Geometry: final body of the model. Coordinates: model frame, mm. A direction names the side the tool comes from. Give positions to 0.01 mm unless a question says otherwise; leave off trailing zeros. Write each loop counter-clockwise with the first axis right and the second up, starting at its lowest first coordinate (ties: lowest second). Pieces come first, ordered by that corner, then holes.
```python
from build123d import *

# Parameters (mm, degrees)
CYLINDER002_R     = 1.5
CYLINDER002_DEPTH = 10
CYLINDER001_R     = 1.5
CYLINDER001_DEPTH = 10
SKETCH_W          = 30
SKETCH_H          = 40
SKETCH_W_2        = 28
SKETCH_H_2        = 38
PAD_DEPTH         = 2
CYLINDER006_R     = 1.8
CYLINDER006_DEPTH = 6
CYLINDER007_R     = 1.8
CYLINDER007_DEPTH = 6
CYLINDER008_R     = 1.8
CYLINDER008_DEPTH = 6
CYLINDER005_R     = 1.8
CYLINDER005_DEPTH = 6
BOX001_W          = 26
BOX001_H          = 36
BOX001_DEPTH      = 17
BOX_W             = 44
BOX_H             = 44
BOX_DEPTH         = 19


with BuildPart() as obj1:
    # Cylinder002 → Cylinder002 (new body)
    with BuildSketch(Plane(origin=(25, 35, 2), x_dir=(1, 0, 0), z_dir=(0, 0, 1))):
        Circle(CYLINDER002_R)
    extrude(amount=CYLINDER002_DEPTH)


with BuildPart() as obj2:
    # Cylinder001 → Cylinder001 (new body)
    with BuildSketch(Plane(origin=(5, 5, 2), x_dir=(1, 0, 0), z_dir=(0, 0, 1))):
        Circle(CYLINDER001_R)
    extrude(amount=CYLINDER001_DEPTH)


with BuildPart() as fusion022:
    # Sketch → Pad (new body)
    with BuildSketch(Plane(origin=(2, 2, 19), x_dir=(1, 0, 0), z_dir=(0, 0, 1))):
        with Locations((13, 18)):
            Rectangle(SKETCH_W, SKETCH_H)
        with Locations((13, 18)):
            Rectangle(SKETCH_W_2, SKETCH_H_2, mode=Mode.SUBTRACT)
    extrude(amount=PAD_DEPTH)

    # Fusion022: union obj1, obj2
    add(obj1.part)
    add(obj2.part)


with BuildPart() as obj3:
    # Cylinder006 → Cylinder006 (new body)
    with BuildSketch(Plane(origin=(-3, 38, 15), x_dir=(1, 0, 0), z_dir=(0, 0, 1))):
        Circle(CYLINDER006_R)
    extrude(amount=CYLINDER006_DEPTH)


with BuildPart() as obj4:
    # Cylinder007 → Cylinder007 (new body)
    with BuildSketch(Plane(origin=(33, 2, 15), x_dir=(1, 0, 0), z_dir=(0, 0, 1))):
        Circle(CYLINDER007_R)
    extrude(amount=CYLINDER007_DEPTH)


with BuildPart() as obj5:
    # Cylinder008 → Cylinder008 (new body)
    with BuildSketch(Plane(origin=(33, 38, 15), x_dir=(1, 0, 0), z_dir=(0, 0, 1))):
        Circle(CYLINDER008_R)
    extrude(amount=CYLINDER008_DEPTH)


with BuildPart() as screw_cut001:
    # Cylinder005 → Cylinder005 (new body)
    with BuildSketch(Plane(origin=(-3, 2, 15), x_dir=(1, 0, 0), z_dir=(0, 0, 1))):
        Circle(CYLINDER005_R)
    extrude(amount=CYLINDER005_DEPTH)

    # Fusion017: union obj3, obj4, obj5
    add(obj3.part)
    add(obj4.part)
    add(obj5.part)


with BuildPart() as box_in:
    # Box001 → Box001 (new body)
    with BuildSketch(Plane(origin=(2, 2, 2), x_dir=(1, 0, 0), z_dir=(0, 0, 1))):
        with Locations((13, 18)):
            Rectangle(BOX001_W, BOX001_H)
    extrude(amount=BOX001_DEPTH)


with BuildPart() as base_final:
    # Box → Box (new body)
    with BuildSketch(Plane(origin=(-7, -2, 0), x_dir=(1, 0, 0), z_dir=(0, 0, 1))):
        with Locations((22, 22)):
            Rectangle(BOX_W, BOX_H)
    extrude(amount=BOX_DEPTH)

    # Cut: cut Box_in
    add(box_in.part, mode=Mode.SUBTRACT)

    # Cut007: cut Screw_cut001
    add(screw_cut001.part, mode=Mode.SUBTRACT)

    # Fusion023: union Fusion022
    add(fusion022.part)


solid = base_final.part
```
Item 1: Reachability of faces 5 (the face through (15, 38, 10)), 6 (the face through (15, -2, 9)), 7 (the face through (15, 40, 20)) from +Z, -Z, +X, -X, +Y, -Y: full face, straight path, thin tool, end or side. Return the list, or none.
Found:
face 5: +Z
face 6: +Z, -Z, +X, -X, -Y
face 7: +Z, +X, -X, +Y
Item 2: Section C-C, the plane x = 33. Return the cut outline in (y, z), plus the area to 3 significant figures.
Found:
outline: (-2, 0) - (42, 0) - (42, 19) - (39.8, 19) - (39.8, 15) - (36.2, 15) - (36.2, 19) - (3.8, 19) - (3.8, 15) - (0.2, 15) - (0.2, 19) - (-2, 19) - close
area: 807 mm2
Item 3: Pin query (flat end, axial travel): pin 1 Ø4 at (x, y) = (-3, 38) entering from +Z; pin 2 Ø3.5 at (x, y) = (4.5, 4.5) entering from +Z; pin 3 Ø1.8 at (x, y) = (-3, 2) entering from +Z; pin 4 Ø10 at (x, y) = (28, 9) entering from +Z. Return the tip coordinate at first contact, or that it passes through.
Found:
pin 1: stops at z = 19
pin 2: stops at z = 12
pin 3: stops at z = 15
pin 4: stops at z = 21
Item 4: Line query: L1, parallel to Y at x = -3, z = 16.8; L2, parallel to X at y = 6, z = 17.75; L3, parallel to Y at x = 25.5, z = 17.25. Output: solid intervals per line, ascending.
Found:
L1: y = -2 to 0.2, 3.8 to 36.2, 39.8 to 42
L2: x = -7 to 2, 28 to 37
L3: y = -2 to 2, 38 to 42
Item 5: Pull-direction query (X, two-part tool) for faces 1 (the face through (-3, 2, 15)), 2 (the face through (30, 20, 20)), 3 (the face through (25, 35, 12)), 4 (the face through (31, 18, 19)); classes: +X half, -X half, draft (parallel to the pull), parting line (faces both ways), or undercut.
Found:
face 1: undercut
face 2: +X half
face 3: undercut
face 4: draft
Item 6: Section A-A, the plane z = 11. Return the cut outline in (x, y), plus the area to 3 significant figures.
Found:
outline: (-7, -2) - (37, -2) - (37, 42) - (-7, 42) - close; circle Ø3 at (5, 5); circle Ø3 at (25, 35); hole (2, 2) - (28, 2) - (28, 38) - (2, 38) - close
area: 1,010 mm2
Item 7: Section D-D, the plane x = 10. Return the cut outline in (y, z), plus the area to 3 significant figures.
Found:
outline: (-2, 0) - (42, 0) - (42, 19) - (40, 19) - (40, 21) - (39, 21) - (39, 19) - (38, 19) - (38, 2) - (2, 2) - (2, 19) - (1, 19) - (1, 21) - (0, 21) - (0, 19) - (-2, 19) - close
area: 228 mm2
Item 8: Section B-B, the plane y = 5. Return the cut outline in (x, z).
Found:
outline: (-7, 0) - (37, 0) - (37, 19) - (30, 19) - (30, 21) - (29, 21) - (29, 19) - (28, 19) - (28, 2) - (6.5, 2) - (6.5, 12) - (3.5, 12) - (3.5, 2) - (2, 2) - (2, 19) - (1, 19) - (1, 21) - (0, 21) - (0, 19) - (-7, 19) - close
